Part print with two shaded views. Sizes in mm from the minimum x, y, z corner. A direction names the side the tool comes from. Give positions to 0.01 mm unless a question says otherwise; leave off trailing zeros. Order: outer loops, then holes, each group sorted by start corner. A loop starts at its lowest first (then second) coordinate and runs counter-clockwise, first axis right, second up. Notation, with made-up numbers: (41.5, 88) - (51.5, 88) arc R17 ccw to (51.5, 112) - close; hole circle Ø1 at (46, -18.5). An arc over 180 degrees is marked (long way). Return JSON: item names as keys, results as strings. Group by question number.
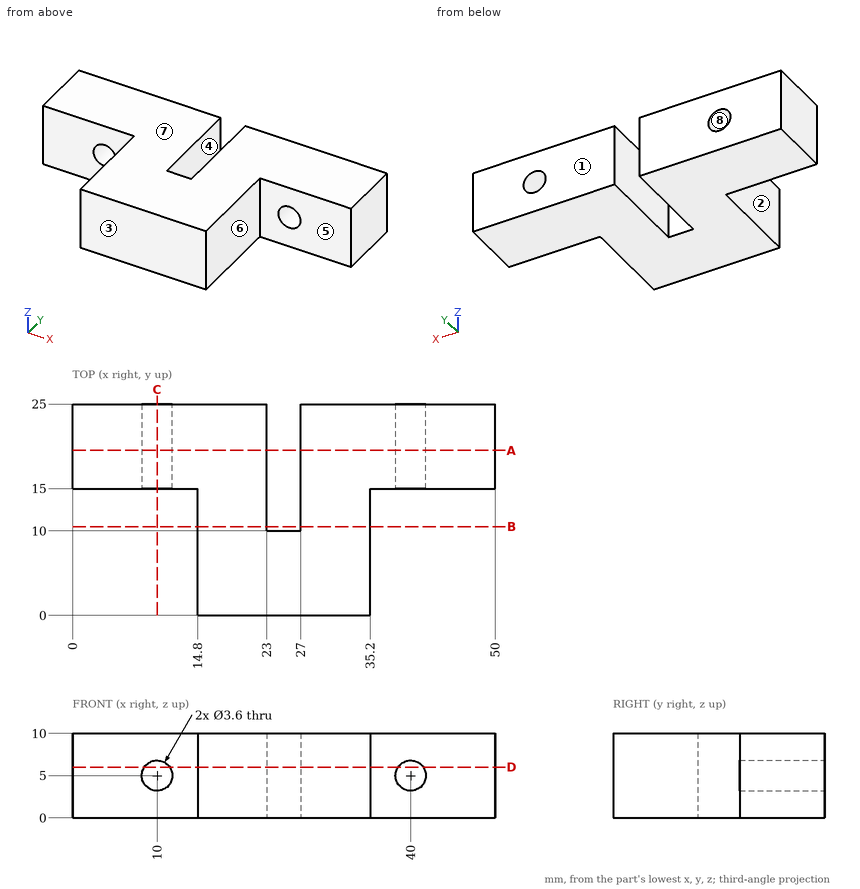
(1) Slice it at C-C (x = 10). Give the cut face in (y, z).
(2) 3-axis set-ups, long thin cutter, end or side, ignore diameter. For the marked faces 1, 2, 3, 4 and 5: which of +Z, -Z, +X, -X, +Y, -Y reach the whole face in a straight line?
(3) Drop flat-ended pins along their axis: pin 1 Ø5 at (x, z) = (42.5, 5.5) entering from -Y; pin 2 Ø3 at (x, z) = (10, 5) entering from -Y. Give the stop position or say it passes through.
(4) Slice it at A-A (y = 19.5). Give the cut face in (x, z), and give its area (3 significant figures).
(5) Slice it at B-B (y = 10.5). Give the cut face in (x, z).
(6) Drill centre lines: L1, parallel to Z at x = 40, y = 20.5; L2, parallel to X at y = 18.5, z = 3.5; L3, parallel to Y at x = 44, z = 6.25. Where is each one in solid material? Low to high.
(7) Pull direction X, two halves, no side cores. Call the marked faces 6, 7 and 8: released by +X, released by -X, zero draft, split by the parting line, or undercut.
(8) Slice it at D-D (z = 6). Give the cut face in (x, y).
Result set:
{
 "1": {"outline": "(15, 0) - (25, 0) - (25, 3.2) - (15, 3.2) - close; (15, 6.8) - (25, 6.8) - (25, 10) - (15, 10) - close"},
 "2": {"face 1": "+Z, -Z, +X, -X, +Y", "face 2": "+Z, -Z, -X, -Y", "face 3": "+Z, -Z, +X, -X, -Y", "face 4": "+Z, -Z, +Y", "face 5": "+Z, -Z, +X, -Y"},
 "3": {"pin 1": "stops at y = 15", "pin 2": "passes through"},
 "4": {"outline": "(0, 0) - (23, 0) - (23, 10) - (0, 10) - close; (27, 0) - (50, 0) - (50, 10) - (27, 10) - close; hole circle Ø3.6 at (10, 5); hole circle Ø3.6 at (40, 5)", "area": "440 mm²"},
 "5": {"outline": "(14.8, 0) - (23, 0) - (23, 10) - (14.8, 10) - close; (27, 0) - (35.2, 0) - (35.2, 10) - (27, 10) - close"},
 "6": {"L1": "z = 0 to 3.2, 6.8 to 10", "L2": "x = 0 to 9.01, 10.99 to 23, 27 to 39.01, 40.99 to 50", "L3": "y = 15 to 25"},
 "7": {"face 6": "released by +X", "face 7": "zero draft", "face 8": "undercut"},
 "8": {"outline": "(0, 15) - (8.5, 15) - (8.5, 25) - (0, 25) - close; (11.5, 15) - (14.8, 15) - (14.8, 0) - (35.2, 0) - (35.2, 15) - (38.5, 15) - (38.5, 25) - (27, 25) - (27, 10) - (23, 10) - (23, 25) - (11.5, 25) - close; (41.5, 15) - (50, 15) - (50, 25) - (41.5, 25) - close"}
}
